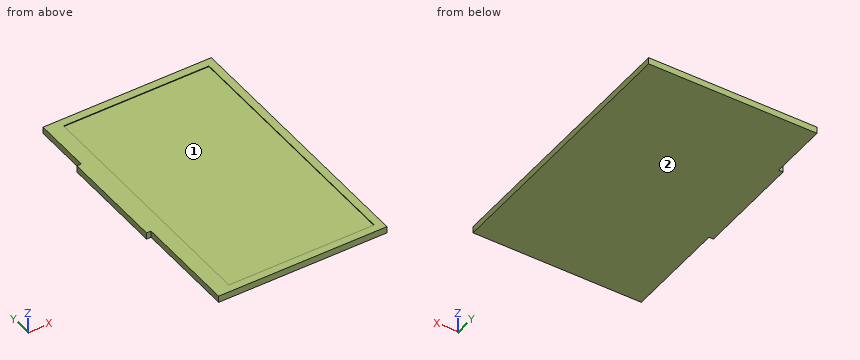
from build123d import *

# Parameters (mm, degrees)
F0_W     = 75.9
F0_H     = 120.9
F1_DEPTH = 3
F2_W     = 65.5
F2_H     = 113.75
F3_DEPTH = 0.3
F4_W     = 48
F4_H     = 3
F5_DEPTH = 2


with BuildPart() as f1:
    # F0 (on Top) → F1 (new body)
    with BuildSketch(Plane.XY):
        with Locations((-2.06492, 0.058994)):
            Rectangle(F0_W, F0_H)
    extrude(amount=F1_DEPTH)

    # F2 (on face) → F3 (cut)
    with BuildSketch(Plane.XY.offset(3)):
        with Locations((-0.36492, -0.016006)):
            Rectangle(F2_W, F2_H)
    extrude(amount=-F3_DEPTH, mode=Mode.SUBTRACT)

    # F4 (on face) → F5 (join)
    with BuildSketch(Plane(origin=(-40.01492, 0, 0), x_dir=(0, -1, 0), z_dir=(-1, 0, 0))):
        with Locations((-10.178994, 1.5)):
            Rectangle(F4_W, F4_H)
    extrude(amount=F5_DEPTH)


solid = f1.part
Verification items for the finished model (mm, model axes). Face numbers are marked on the shaded views. Coordinates: 2 decimals unless noted, no trailing zeros. Order: outer loops, then holes, each group sorted by start corner. A loop starts at its lowest first (then second) coordinate and runs counter-clockwise, first axis right, second up. Notation, with made-up numbers: (-21, -22) -> (14, -22) arc R18 ccw to (14, -8) -> close; hole circle Ø2 at (86.25, -11.75). An arc over 180 degrees is marked (long way). Put each result on its own line as item: value. Start each with the question number.
1. Material ranges on L1, parallel to X at y = -5, z = 2.95; L2, parallel to X at y = 39, z = 2.9; L3, parallel to Z at x = -22.5, y = -2, recorded low to high. Write a range as [from, to].
2. Cross-section at A-A, the plane z = 1.8. Record the boundary of the cut face in (x, y), then the cut area to 3 significant figures.
3. Go/stop test with flat-tipped pins: pin 1 Ø8 at (x, y) = (-25, 25) entering from +Z; pin 2 Ø4 at (x, y) = (-2.5, -22.5) entering from -Z; pin 3 Ø1.5 at (y, z) = (51.5, 1.5) entering from -X; pin 4 Ø0.6 at (x, z) = (-41.5, 1.5) entering from +Y. Record where each tip stops, or that it passes through.
4. Mould release check, pull along Y, two halves, no side actions. Record for the marked faces 1 and 2: released by +Y, released by -Y, zero draft, split by the parting line, or undercut.
5. Cross-section at B-B, the plane y = -32.5. Record the boundary of the cut face in (x, z), then the cut area to 3 significant figures.
Computed:
1. L1: [-42.01, -33.11], [32.39, 35.89]
1. L2: [-40.01, -33.11], [32.39, 35.89]
1. L3: [0, 2.7]
2. outline: (-42.01, -13.82) -> (-40.01, -13.82) -> (-40.01, -60.39) -> (35.89, -60.39) -> (35.89, 60.51) -> (-40.01, 60.51) -> (-40.01, 34.18) -> (-42.01, 34.18) -> close
2. area: 9,270 mm2
3. pin 1: z = 2.7
3. pin 2: z = 0
3. pin 3: x = -40.01
3. pin 4: y = 34.18
4. face 1: undercut
4. face 2: zero draft
5. outline: (-40.01, 0) -> (35.89, 0) -> (35.89, 3) -> (32.39, 3) -> (32.39, 2.7) -> (-33.11, 2.7) -> (-33.11, 3) -> (-40.01, 3) -> close
5. area: 208 mm2
